```python
from build123d import *

# Parameters (mm, degrees)
SKETCH1_W                                            = 2.925965508
SKETCH1_H                                            = 4.901580006
BOSS_EXTRUDE1_DEPTH                                  = 2
CSK_FOR_M2_FLAT_HEAD_MACHINE_SCREW2_D                = 2.4
CSK_FOR_M2_FLAT_HEAD_MACHINE_SCREW2_DEPTH            = 42.93
CSK_FOR_M2_FLAT_HEAD_MACHINE_SCREW2_CSINK_D          = 3.5
CSK_FOR_M2_FLAT_HEAD_MACHINE_SCREW2_CSINK_ANGLE      = 90
CSK_FOR_M2_FLAT_HEAD_MACHINE_SCREW2_TIP              = 0.721032743
CSK_FOR_M2_CROSS_COUNTERSUNK_HEAD_SCREW1_D           = 2.75
CSK_FOR_M2_CROSS_COUNTERSUNK_HEAD_SCREW1_DEPTH       = 8.7
CSK_FOR_M2_CROSS_COUNTERSUNK_HEAD_SCREW1_CSINK_D     = 4
CSK_FOR_M2_CROSS_COUNTERSUNK_HEAD_SCREW1_CSINK_ANGLE = 92
CSK_FOR_M2_CROSS_COUNTERSUNK_HEAD_SCREW1_TIP         = 0.826183351
CUT_EXTRUDE1_DEPTH                                   = 1.5


with BuildPart() as part:
    # Sketch1 → Boss-Extrude1 (new body)
    with BuildSketch(Plane(origin=(0, 0, 0), x_dir=(1, 0, 0), z_dir=(0, 1, 0))):
        Polygon((-11.293051345, 29.704532022), (12.706948655, 29.704532022), (15.706948655, 26.704532022), (15.706948655, 2.704532022), (12.706948655, -0.295467978), (-11.293051345, -0.295467978), (-14.293051345, 2.704532022), (-14.293051345, 26.704532022), align=None)
        with Locations((0.743965901, 16.189415938)):
            Rectangle(SKETCH1_W, SKETCH1_H, mode=Mode.SUBTRACT)
    extrude(amount=BOSS_EXTRUDE1_DEPTH)

    # CSK for M2 Flat Head Machine Screw2
    with Locations(Plane(origin=(0, 2, 0), x_dir=(1, 0, 0), z_dir=(0, 1, 0))):
        with Locations((-11.293051345, 26.704532022), (-11.293051345, 2.704532022), (12.706948655, 26.704532022), (12.706948655, 2.704532022)):
            CounterSinkHole(CSK_FOR_M2_FLAT_HEAD_MACHINE_SCREW2_D / 2, CSK_FOR_M2_FLAT_HEAD_MACHINE_SCREW2_CSINK_D / 2, depth=CSK_FOR_M2_FLAT_HEAD_MACHINE_SCREW2_DEPTH, counter_sink_angle=CSK_FOR_M2_FLAT_HEAD_MACHINE_SCREW2_CSINK_ANGLE)
            with Locations((0, 0, -(CSK_FOR_M2_FLAT_HEAD_MACHINE_SCREW2_DEPTH + CSK_FOR_M2_FLAT_HEAD_MACHINE_SCREW2_TIP / 2))):  # 118° drill point
                Cone(0, CSK_FOR_M2_FLAT_HEAD_MACHINE_SCREW2_D / 2, CSK_FOR_M2_FLAT_HEAD_MACHINE_SCREW2_TIP, mode=Mode.SUBTRACT)

    # CSK for M2 Cross Countersunk Head Screw1
    with Locations(Plane.XZ):
        with Locations((-3.793051345, -14.704532022), (5.206948655, -14.704532022)):
            CounterSinkHole(CSK_FOR_M2_CROSS_COUNTERSUNK_HEAD_SCREW1_D / 2, CSK_FOR_M2_CROSS_COUNTERSUNK_HEAD_SCREW1_CSINK_D / 2, depth=CSK_FOR_M2_CROSS_COUNTERSUNK_HEAD_SCREW1_DEPTH, counter_sink_angle=CSK_FOR_M2_CROSS_COUNTERSUNK_HEAD_SCREW1_CSINK_ANGLE)
            with Locations((0, 0, -(CSK_FOR_M2_CROSS_COUNTERSUNK_HEAD_SCREW1_DEPTH + CSK_FOR_M2_CROSS_COUNTERSUNK_HEAD_SCREW1_TIP / 2))):  # 118° drill point
                Cone(0, CSK_FOR_M2_CROSS_COUNTERSUNK_HEAD_SCREW1_D / 2, CSK_FOR_M2_CROSS_COUNTERSUNK_HEAD_SCREW1_TIP, mode=Mode.SUBTRACT)

    # Sketch11 → Cut-Extrude1 (cut)
    with BuildSketch(Plane(origin=(0, 2, 0), x_dir=(1, 0, 0), z_dir=(0, 1, 0))):
        with BuildLine():
            Line((-5.293051345, 24.204532022), (-5.293051345, 14.704532022))
            ThreePointArc((-5.293051345, 14.704532022), (-4.853711517, 13.64387185), (-3.793051345, 13.204532022))
            Line((-3.793051345, 13.204532022), (5.206948655, 13.204532022))
            ThreePointArc((5.206948655, 13.204532022), (6.267608827, 13.64387185), (6.706948655, 14.704532022))
            Line((6.706948655, 14.704532022), (6.706948655, 24.204532022))
            ThreePointArc((6.706948655, 24.204532022), (6.414055436, 24.911638803), (5.706948655, 25.204532022))
            Line((5.706948655, 25.204532022), (-4.293051345, 25.204532022))
            ThreePointArc((-4.293051345, 25.204532022), (-5.000158126, 24.911638803), (-5.293051345, 24.204532022))
        make_face()
    extrude(amount=-CUT_EXTRUDE1_DEPTH, mode=Mode.SUBTRACT)


solid = part.part
```
Part model, mm, in its own coordinate system. A direction names the side the tool comes from. Round coordinates to 2 decimals unless told otherwise and drop trailing zeros. Order: outer loops, then holes, each group sorted by start corner. A loop starts at its lowest first (then second) coordinate and runs counter-clockwise, first axis right, second up. Notation, with made-up numbers: M 74,-14 L 97,-14 A20 cw 97,2 Z; hole C 14,48 d2. An arc over 180 degrees is marked long. Answer in a Markdown table with one row per item. Add a question column.
Q1. 3-axis set-ups, long thin cutter, end or side, ignore diameter. For faces 1 (the face through (1, 1, -25.205)), 2 (the face through (1, 2, -12)): which of +Z, -Z, +X, -X, +Y, -Y reach the whole face in a straight line?
Q2. Cut at A-A on z = -19.25. Give the cut face in (x, y), and give its area (3 significant figures).
Q3. Wall check: L1, parallel to X at y = 0.8, z = -15.5; L2, parallel to Z at x = 13, y = 1.45; L3, parallel to Y at x = -2.5, z = -20.75. Give the ranges that are in metal, low to high. Write a range as from..to.
Q4. Mould opens along X. For faces 3 (the face through (1, 1, -29.705)), 4 (the face through (6.707, 1, -19)), 5 (the face through (-12.77, 0.99, -1.18)) say: +X half, -X half, draft (parallel to the pull), parting line (faces both ways), or undercut.
Q5. Pin check, flat tips, straight feed: pin 1 (2 mm diameter, centred on x = 12.71, z = -2.7, fed in from -Y); pin 2 (3 mm diameter, centred on x = -11.29, z = -2.7, fed in from +Y). Stop position of each tip, or through.
Q6. Cut at B-B on x = -10.5. Give the number of separate pieces and of enclosed holes in the cut face, and give its area (4 significant figures).
Established:
| question | item | result |
|---|---|---|
| 1 | face 1 | +Y |
| 1 | face 2 | +Z, -Z, +X, -X, +Y |
| 2 | outline | M -14.29,0 L 15.71,0 L 15.71,2 L 6.71,2 L 6.71,0.5 L -5.29,0.5 L -5.29,2 L -14.29,2 Z |
| 2 | area | 42.0 mm2 |
| 3 | L1 | x = -14.29..-5.29, 6.71..15.71 |
| 3 | L2 | z = -29.41..-27.87, -25.54..-3.87, -1.54..0 |
| 3 | L3 | y = 0..0.5 |
| 4 | face 3 | draft |
| 4 | face 4 | undercut |
| 4 | face 5 | -X half |
| 5 | pin 1 | passes through |
| 5 | pin 2 | stops at y = 1.76 |
| 6 | separate pieces | 3 |
| 6 | enclosed holes | 0 |
| 6 | area | 52.05 mm2 |
